from build123d import *

# Parameters (mm, degrees)
ESBO_O1_W                = 195
ESBO_O1_H                = 195
RESSALTO_EXTRUS_O1_DEPTH = 10
ESBO_O2_W                = 7
ESBO_O2_H                = 32
ESBO_O2_W_2              = 32
ESBO_O2_H_2              = 7
CORTE_EXTRUS_O1_DEPTH    = 11
ESBO_O3_W                = 6.3
ESBO_O3_H                = 195
CORTE_EXTRUS_O2_DEPTH    = 4
ESBO_O4_R                = 1.5
CORTE_EXTRUS_O3_DEPTH    = 11
ESBO_O5_R                = 1.5
CORTE_EXTRUS_O4_DEPTH    = 11
ESBO_O6_W                = 5
ESBO_O6_H                = 2.5
ESBO_O6_H_2              = 5
ESBO_O6_W_2              = 2.5
RESSALTO_EXTRUS_O2_DEPTH = 5


with BuildPart() as part:
    # Esboço1 → Ressalto-extrusão1 (new body)
    with BuildSketch(Plane(origin=(0, 0, 0), x_dir=(1, 0, 0), z_dir=(0, 1, 0))):
        Rectangle(ESBO_O1_W, ESBO_O1_H)
    extrude(amount=RESSALTO_EXTRUS_O1_DEPTH)

    # Esboço2 → Corte-extrusão1 (cut, through all)
    with BuildSketch(Plane(origin=(0, 10, 0), x_dir=(1, 0, 0), z_dir=(0, 1, 0))):
        with Locations((-87.5, 47.5)):
            Rectangle(ESBO_O2_W, ESBO_O2_H)
        with Locations((-87.5, -47.5)):
            Rectangle(ESBO_O2_W, ESBO_O2_H)
        with Locations((-27.5, -92.5)):
            Rectangle(ESBO_O2_W_2, ESBO_O2_H_2)
        with Locations((47.5, -92.5)):
            Rectangle(ESBO_O2_W_2, ESBO_O2_H_2)
        with Locations((47.5, 92.5)):
            Rectangle(ESBO_O2_W_2, ESBO_O2_H_2)
        with Locations((-27.5, 92.5)):
            Rectangle(ESBO_O2_W_2, ESBO_O2_H_2)
    extrude(amount=-CORTE_EXTRUS_O1_DEPTH, mode=Mode.SUBTRACT)

    # Esboço3 → Corte-extrusão2 (cut)
    with BuildSketch(Plane(origin=(0, 10, 0), x_dir=(1, 0, 0), z_dir=(0, 1, 0))):
        with Locations((89.35, 0)):
            Rectangle(ESBO_O3_W, ESBO_O3_H)
    extrude(amount=-CORTE_EXTRUS_O2_DEPTH, mode=Mode.SUBTRACT)

    # Esboço4 → Corte-extrusão3 (cut, through all)
    with BuildSketch(Plane.XZ):
        with Locations((-87.5, 92.5)):
            Circle(ESBO_O4_R)
        with Locations((-87.5, -92.5)):
            Circle(ESBO_O4_R)
    extrude(amount=-CORTE_EXTRUS_O3_DEPTH, mode=Mode.SUBTRACT)

    # Esboço5 → Corte-extrusão4 (cut, through all)
    with BuildSketch(Plane.XZ):
        with Locations((75, 92.5)):
            Circle(ESBO_O5_R)
        with Locations((75, -92.5)):
            Circle(ESBO_O5_R)
    extrude(amount=-CORTE_EXTRUS_O4_DEPTH, mode=Mode.SUBTRACT)

    # Esboço6 → Ressalto-extrusão2 (add)
    with BuildSketch(Plane(origin=(0, 10, 0), x_dir=(1, 0, 0), z_dir=(0, 1, 0))):
        with Locations((10, -3.75)):
            Rectangle(ESBO_O6_W, ESBO_O6_H)
        with Locations((10, 0)):
            Rectangle(ESBO_O6_W, ESBO_O6_H_2)
        with Locations((13.75, 0)):
            Rectangle(ESBO_O6_W_2, ESBO_O6_H_2)
        with Locations((6.25, 0)):
            Rectangle(ESBO_O6_W_2, ESBO_O6_H_2)
        with Locations((10, 3.75)):
            Rectangle(ESBO_O6_W, ESBO_O6_H)
    extrude(amount=RESSALTO_EXTRUS_O2_DEPTH)


solid = part.part
Verification items for the finished model (mm, model axes). A direction names the side the tool comes from. Round coordinates to 2 decimals unless told otherwise and drop trailing zeros. Loops run counter-clockwise (first coordinate to the right, second up) from the corner with the lowest first, then second, coordinate; pieces in that order, holes last. Notation, with made-up numbers: (39.5, 69) - (62.5, 69) arc R10 ccw to (62.5, 74) - close; hole circle Ø7 at (11.25, -33.5). An arc over 180 degrees is marked (long way). Answer in a Markdown table with one row per item. Add a question column.
Q1. Material ranges on line 1 (Z direction, x = -87.5, y = 7.75); line 2 (X direction, y = 7.25, z = 92.5); line 3 (X direction, y = 4.25, z = -92.5), recorded low to high.
Q2. Section check D-D on x = 66. Enter the section's corners in (y, z), plus the area to 3 significant figures.
Q3. Tool access check on faces 1 (the face through (89, 6, -1)), 2 (the face through (-28, 5, -89)), 3 (the face through (15, 12, 0)), 4 (the face through (-1, 5, -97.5)). Record the directions out of +Z, -Z, +X, -X, +Y, -Y that give a thin tool (end or side, any length) a straight path to the whole face; none if there is none.
Q4. Release check for a two-part mould opening along Z. For faces 5 (the face through (-1, 0, -1)), 6 (the face through (10, 12, 5)), 7 (the face through (-84, 5, 48)) record: pulls with the +Z half, pulls with the -Z half, needs draft (parallel to the pull), parting line crosses it, or undercut.
Q5. Section check B-B on x = -35. Enter the section's corners in (y, z).
Q6. Section check C-C on z = -85. Enter the section's corners in (x, y).
Q7. Gauge pin test, flat ends, axial feed: pin 1 (5.5 mm diameter, centred on y = 13.5, z = 0.5, fed in from +X); pin 2 (0.8 mm diameter, centred on y = 11.5, z = -3.5, fed in from -X); pin 3 (4 mm diameter, centred on x = -87.5, z = -92.5, fed in from +Y). Record the tip position at first contact, or that the pin passes through.
Q8. Section check A-A on z = 36. Enter the section's corners in (x, y), plus the area to 3 significant figures.
Found:
| question | item | result |
|---|---|---|
| 1 | line 1 | z = -97.5 to -94, -91 to -63.5, -31.5 to 31.5, 63.5 to 91, 94 to 97.5 |
| 1 | line 2 | x = -97.5 to -89, -86 to -43.5, -11.5 to 31.5, 63.5 to 73.5, 76.5 to 86.2, 92.5 to 97.5 |
| 1 | line 3 | x = -97.5 to -89, -86 to -43.5, -11.5 to 31.5, 63.5 to 73.5, 76.5 to 97.5 |
| 2 | outline | (0, -97.5) - (10, -97.5) - (10, 97.5) - (0, 97.5) - close |
| 2 | area | 1,950 mm² |
| 3 | face 1 | +Z, -Z, +Y |
| 3 | face 2 | +Y, -Y |
| 3 | face 3 | +Z, -Z, +X, +Y |
| 3 | face 4 | -Z, +X, -X, +Y, -Y |
| 4 | face 5 | needs draft |
| 4 | face 6 | pulls with the +Z half |
| 4 | face 7 | undercut |
| 5 | outline | (0, -97.5) - (10, -97.5) - (10, -96) - (0, -96) - close; (0, -89) - (10, -89) - (10, 89) - (0, 89) - close; (0, 96) - (10, 96) - (10, 97.5) - (0, 97.5) - close |
| 6 | outline | (-97.5, 0) - (97.5, 0) - (97.5, 10) - (92.5, 10) - (92.5, 6) - (86.2, 6) - (86.2, 10) - (-97.5, 10) - close |
| 7 | pin 1 | stops at x = 15 |
| 7 | pin 2 | stops at x = 7.5 |
| 7 | pin 3 | stops at y = 10 |
| 8 | outline | (-97.5, 0) - (-91, 0) - (-91, 10) - (-97.5, 10) - close; (-84, 0) - (97.5, 0) - (97.5, 10) - (92.5, 10) - (92.5, 6) - (86.2, 6) - (86.2, 10) - (-84, 10) - close |
| 8 | area | 1,850 mm² |
